CAD build for the part. Positions are in the model's coordinates, mm. Face numbers are marked on the shaded views. Give positions to 0.01 mm unless a question says otherwise; leave off trailing zeros. Loops run counter-clockwise (first coordinate to the right, second up) from the corner with the lowest first, then second, coordinate; pieces in that order, holes last.
```python
from build123d import *

# Parameters (mm, degrees)
SKETCH1_W           = 25
SKETCH1_H           = 20
BOSS_EXTRUDE1_DEPTH = 3
SKETCH2_W           = 3
SKETCH2_H           = 20
BOSS_EXTRUDE2_DEPTH = 4
SKETCH3_W           = 25
SKETCH3_H           = 20
BOSS_EXTRUDE3_DEPTH = 4


with BuildPart() as part:
    # Sketch1 → Boss-Extrude1 (new body)
    with BuildSketch(Plane(origin=(0, 0, 0), x_dir=(1, 0, 0), z_dir=(0, 1, 0))):
        with Locations((12.5, 10)):
            Rectangle(SKETCH1_W, SKETCH1_H)
    extrude(amount=BOSS_EXTRUDE1_DEPTH)

    # Sketch2 → Boss-Extrude2 (add)
    with BuildSketch(Plane(origin=(0, 3, 0), x_dir=(1, 0, 0), z_dir=(0, 1, 0))):
        with Locations((1.5, 10)):
            Rectangle(SKETCH2_W, SKETCH2_H)
        with Locations((23.5, 10)):
            Rectangle(SKETCH2_W, SKETCH2_H)
    extrude(amount=BOSS_EXTRUDE2_DEPTH)

    # Sketch3 → Boss-Extrude3 (add)
    with BuildSketch(Plane(origin=(0, 7, 0), x_dir=(1, 0, 0), z_dir=(0, 1, 0))):
        with Locations((12.5, 10)):
            Rectangle(SKETCH3_W, SKETCH3_H)
    extrude(amount=BOSS_EXTRUDE3_DEPTH)


solid = part.part
```
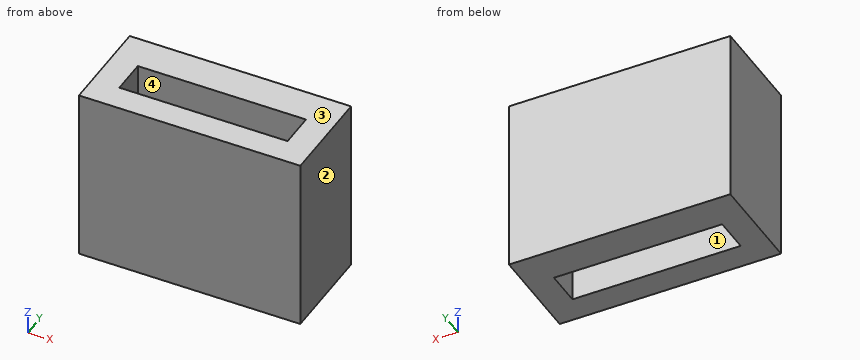
1. Saw through at B-B, the plane y = 3.5. List the corners of the cut face in (x, z).
Responses:
outline: (0, -20) - (3, -20) - (3, 0) - (0, 0) - close; (22, -20) - (25, -20) - (25, 0) - (22, 0) - close
2. Saw through at A-A, the plane x = 19. List the corners of the cut face in (y, z).
Responses:
outline: (0, -20) - (3, -20) - (3, 0) - (0, 0) - close; (7, -20) - (11, -20) - (11, 0) - (7, 0) - close
3. Pull direction X, two halves, no side cores. Call the marked faces 1, 2, 3 and 4: released by +X, released by -X, zero draft, split by the parting line, or undercut.
Responses:
face 1: undercut
face 2: released by +X
face 3: zero draft
face 4: undercut
4. Drop a flat-ended pin along its axis: pin 1 (5.5 mm diameter, centred on x = 13, z = -12.5, fed in from -Y). Give the stop position or say it passes through.
Responses:
pin 1: stops at y = 0
5. Probe line 1 along Y through (x, z) = (20.25, -13.5); line 2 along X through (y, z) = (4.25, -7). List the from-to ranges inside material, lowest first.
Responses:
line 1: y = 0 to 3, 7 to 11
line 2: x = 0 to 3, 22 to 25
6. Saw through at C-C, the plane z = -3. List the corners of the cut face in (x, y), and give its area (3 significant figures).
Responses:
outline: (0, 0) - (25, 0) - (25, 11) - (0, 11) - close; hole (3, 3) - (22, 3) - (22, 7) - (3, 7) - close
area: 199 mm2
